Study the drawing (mm; zero at the part's minimum x, y, z) and answer. Give positions to 0.01 mm unless a question says otherwise; leave off trailing zeros. Write each loop counter-clockwise with the first axis right and the second up, starting at its lowest first coordinate (ties: lowest second). Pieces come first, ordered by that corner, then holes. Notation, with made-up numbers: (-37, -24) - (-3, -24) arc R19 cw to (-3, -20) - close; hole circle Ø3 at (-14, -8). An arc over 180 degrees is marked (long way). Return JSON: item names as keys, results as strings.
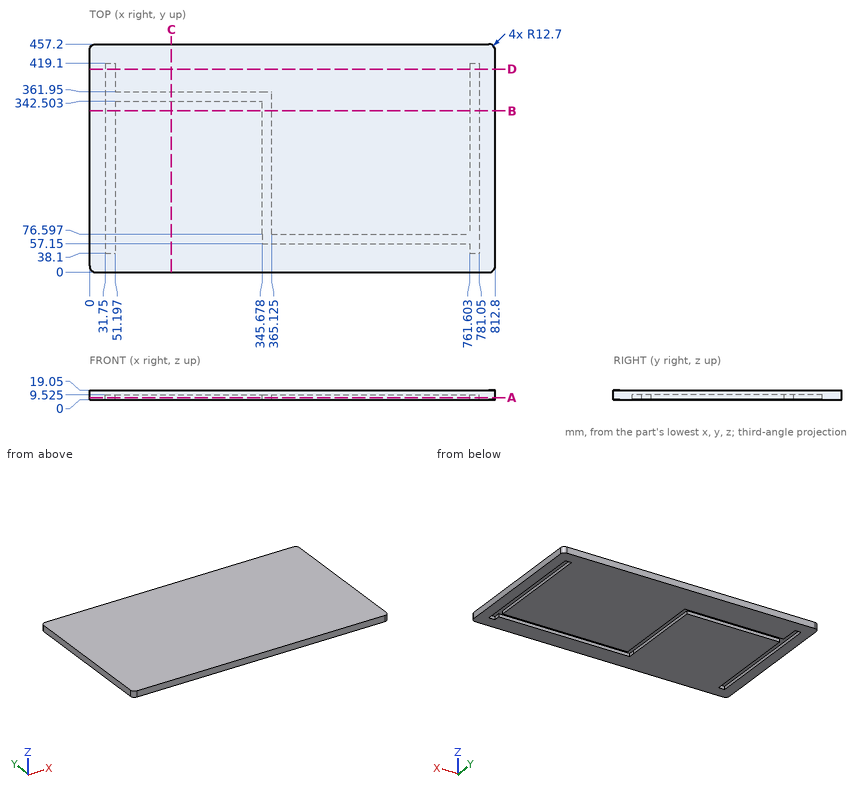
Item 1: Consider L1, parallel to X at y = 398, z = 7; L2, parallel to X at y = 103, z = 3.5 (3 decimals); L3, parallel to X at y = 66.5, z = 4.25. Determine where each line is inside the solid, lowest interval first.
Answer below:
{"L1": "x = 0 to 31.75, 51.2 to 761.6, 781.05 to 812.8", "L2": "x = 0 to 31.75, 51.197 to 345.678, 365.125 to 761.603, 781.05 to 812.8", "L3": "x = 0 to 31.75, 51.2 to 345.68, 781.05 to 812.8"}
Item 2: A cutting plane is placed at A-A on z = 4.25. Determine the outline of the cut face in (x, y) (3 decimals), then the cut area to 3 significant figures.
Answer below:
{"outline": "(0, 12.7) arc R12.7 ccw to (12.7, 0) - (800.1, 0) arc R12.7 ccw to (812.8, 12.7) - (812.8, 444.5) arc R12.7 ccw to (800.1, 457.2) - (12.7, 457.2) arc R12.7 ccw to (0, 444.5) - close; hole (31.75, 38.1) - (51.197, 38.1) - (51.197, 342.503) - (345.678, 342.503) - (345.678, 57.15) - (761.603, 57.15) - (761.603, 38.1) - (781.05, 38.1) - (781.05, 419.1) - (761.603, 419.1) - (761.603, 76.597) - (365.125, 76.597) - (365.125, 361.95) - (51.197, 361.95) - (51.197, 419.1) - (31.75, 419.1) - close", "area": "337,000 mm²"}
Item 3: A cutting plane is placed at D-D on y = 407. Determine the outline of the cut face in (x, z) (3 decimals), then the cut area to 3 significant figures.
Answer below:
{"outline": "(0, 0) - (31.75, 0) - (31.75, 9.525) - (51.197, 9.525) - (51.197, 0) - (761.603, 0) - (761.603, 9.525) - (781.05, 9.525) - (781.05, 0) - (812.8, 0) - (812.8, 19.05) - (0, 19.05) - close", "area": "15,100 mm²"}
Item 4: A cutting plane is placed at C-C on x = 164. Determine the outline of the cut face in (y, z) (3 decimals).
Answer below:
{"outline": "(0, 0) - (342.503, 0) - (342.503, 9.525) - (361.95, 9.525) - (361.95, 0) - (457.2, 0) - (457.2, 19.05) - (0, 19.05) - close"}
Item 5: A cutting plane is placed at B-B on y = 323. Determine the outline of the cut face in (x, z) (3 decimals).
Answer below:
{"outline": "(0, 0) - (31.75, 0) - (31.75, 9.525) - (51.197, 9.525) - (51.197, 0) - (345.678, 0) - (345.678, 9.525) - (365.125, 9.525) - (365.125, 0) - (761.603, 0) - (761.603, 9.525) - (781.05, 9.525) - (781.05, 0) - (812.8, 0) - (812.8, 19.05) - (0, 19.05) - close"}
